Work out the finished part from the listing and answer in its coordinate system (mm). A direction names the side the tool comes from. Round coordinates to 2 decimals unless told otherwise and drop trailing zeros. Write each loop counter-clockwise with the first axis right and the second up, starting at its lowest first coordinate (ties: lowest second). Pieces come first, ordered by that corner, then holes. Notation, with made-up numbers: M 5,7 L 40,7 A31 cw 40,40 Z; hole C 24.5,59.5 d10. An arc over 180 degrees is marked long. Answer in a Markdown table with one row per item.
```python
from build123d import *

# Parameters (mm, degrees)
SKETCH1_W           = 50
SKETCH1_H           = 50
BOSS_EXTRUDE1_DEPTH = 10
SKETCH2_W           = 40
SKETCH2_H           = 20
BOSS_EXTRUDE2_DEPTH = 50
SKETCH3_R           = 3.5
CUT_EXTRUDE1_DEPTH  = 10
SKETCH4_R           = 3
CUT_EXTRUDE2_DEPTH  = 46
SKETCH5_R           = 3.5
CUT_EXTRUDE3_DEPTH  = 10


with BuildPart() as part:
    # Sketch1 → Boss-Extrude1 (new body)
    with BuildSketch(Plane.XY):
        Rectangle(SKETCH1_W, SKETCH1_H)
    extrude(amount=BOSS_EXTRUDE1_DEPTH)

    # Sketch2 → Boss-Extrude2 (add)
    with BuildSketch(Plane.XY.offset(10)):
        Rectangle(SKETCH2_W, SKETCH2_H)
    extrude(amount=BOSS_EXTRUDE2_DEPTH)

    # Sketch3 → Cut-Extrude1 (cut)
    with BuildSketch(Plane.XY.offset(10)):
        with Locations((-18, 18)):
            Circle(SKETCH3_R)
        with Locations((18, 18)):
            Circle(SKETCH3_R)
        with Locations((18, -18)):
            Circle(SKETCH3_R)
        with Locations((-18, -18)):
            Circle(SKETCH3_R)
    extrude(amount=-CUT_EXTRUDE1_DEPTH, mode=Mode.SUBTRACT)

    # Sketch4 → Cut-Extrude2 (cut, through all)
    with BuildSketch(Plane(origin=(20, 0, 0), x_dir=(0, 0, -1), z_dir=(1, 0, 0))):
        with Locations((-35.289984846, 0)):
            Circle(SKETCH4_R)
    extrude(amount=-CUT_EXTRUDE2_DEPTH, mode=Mode.SUBTRACT)

    # Sketch5 → Cut-Extrude3 (cut)
    with BuildSketch(Plane(origin=(0, 10, 0), x_dir=(1, 0, 0), z_dir=(0, 1, 0))):
        with Locations((0, -35.211614701)):
            Circle(SKETCH5_R)
    extrude(amount=-CUT_EXTRUDE3_DEPTH, mode=Mode.SUBTRACT)


solid = part.part
```
1. Given pin 1 (20 mm diameter, centred on x = 0.5, z = 31.5, fed in from +Y); pin 2 (16 mm diameter, centred on y = 0, z = 28, fed in from +X); pin 3 (8 mm diameter, centred on x = -0.5, y = -16.5, fed in from +Z), each flat-ended and moving along its own axis, determine where each tip first touches the part or whether it passes through.
Calculated:
| item | result |
|---|---|
| pin 1 | stops at y = 10 |
| pin 2 | stops at x = 20 |
| pin 3 | stops at z = 10 |
2. The part is cut by section A-A (x = -15.5). Determine the outline of the cut face in (y, z), plus the area to 3 significant figures.
Calculated:
| item | result |
|---|---|
| outline | M -25,0 L -20.45,0 L -20.45,10 L -25,10 Z; M -15.55,0 L 15.55,0 L 15.55,10 L 10,10 L 10,60 L -10,60 L -10,10 L -15.55,10 Z; M 20.45,0 L 25,0 L 25,10 L 20.45,10 Z; hole C 0,35.29 d6 |
| area | 1,370 mm² |
3. A tool of negligible diameter and unlimited length cuts with its end or side. For faces 5 (the flat face through (4, 10, 35)), 6 (the flat face through (-20, 4, 35)), 7 (the flat face through (0, -25, 5)), 8 (the flat face through (0, -10, 35)), 9 (the flat face through (0, 25, 5)), from which of +Z, -Z, +X, -X, +Y, -Y can it reach the whole face along a straight path? Write none if from no direction.
Calculated:
| item | result |
|---|---|
| face 5 | +Z, +X, -X, +Y |
| face 6 | +Z, -X, +Y, -Y |
| face 7 | +Z, -Z, +X, -X, -Y |
| face 8 | +Z, +X, -X, -Y |
| face 9 | +Z, -Z, +X, -X, +Y |
4. The part is cut by section B-B (y = -18). Determine the outline of the cut face in (x, z).
Calculated:
| item | result |
|---|---|
| outline | M -25,0 L -21.5,0 L -21.5,10 L -25,10 Z; M -14.5,0 L 14.5,0 L 14.5,10 L -14.5,10 Z; M 21.5,0 L 25,0 L 25,10 L 21.5,10 Z |
5. Determine the mould class of faces 1 (the flat face through (0, 0, 0)), 2 (the flat face through (20, 4, 35)), 3 (the cylindrical face through (3.34, 6.18, 34.16)), 4 (the cylindrical face through (0.28, -2.93, 35.94)) for opening direction Z: released by +Z, released by -Z, zero draft, split by the parting line, or undercut.
Calculated:
| item | result |
|---|---|
| face 1 | released by -Z |
| face 2 | zero draft |
| face 3 | undercut |
| face 4 | undercut |
6. The part is cut by section D-D (x = 0). Determine the outline of the cut face in (y, z), plus the area to 3 significant figures.
Calculated:
| item | result |
|---|---|
| outline | M -25,0 L 25,0 L 25,10 L 10,10 L 10,31.71 L 0,31.71 L 0,32.29 A3 cw 0,38.29 L 0,38.71 L 10,38.71 L 10,60 L -10,60 L -10,10 L -25,10 Z |
| area | 1,420 mm² |
7. Consider line 1 along Y through (x, z) = (-18, 7.25); line 2 along Z through (x, y) = (-4, 0); line 3 along Y through (x, z) = (-1, 15.5). Determine where each line is inside the solid, lowest interval first. Write a range as from..to.
Calculated:
| item | result |
|---|---|
| line 1 | y = -25..-21.5, -14.5..14.5, 21.5..25 |
| line 2 | z = 0..32.29, 38.29..60 |
| line 3 | y = -10..10 |
8. The part is cut by section C-C (y = -6.5). Determine the outline of the cut face in (x, z), plus the area to 3 significant figures.
Calculated:
| item | result |
|---|---|
| outline | M -25,0 L 25,0 L 25,10 L 20,10 L 20,60 L -20,60 L -20,10 L -25,10 Z |
| area | 2,500 mm² |
